Check sheet for the modelled part. Datum: model origin and axes. Units: mm. A direction names the side the tool comes from. Round coordinates to 2 decimals unless told otherwise and drop trailing zeros. Write each loop counter-clockwise with the first axis right and the second up, starting at its lowest first coordinate (ties: lowest second). Pieces come first, ordered by that corner, then holes.
from build123d import *

# Parameters (mm, degrees)
SKETCH_W             = 33
SKETCH_H             = 90.6
PAD_DEPTH            = 2
SKETCH001_W          = 31.55
SKETCH001_H          = 90.6
PAD001_DEPTH         = 14
SKETCH002_W          = 27.5
SKETCH002_H          = 72.5
POCKET_DEPTH         = 12.001
SKETCH003_W          = 19.5
SKETCH003_H          = 7.2
POCKET001_DEPTH      = 2.001
POCKET001_DEPTH_BACK = -12.001
SKETCH004_R          = 3.25
POCKET002_DEPTH      = 2
FILLET_R             = 2
FILLET001_R          = 1


with BuildPart() as part:
    # Sketch → Pad (new body)
    with BuildSketch(Plane.XY):
        with Locations((43.35, -0.5)):
            Rectangle(SKETCH_W, SKETCH_H)
    extrude(amount=PAD_DEPTH)

    # Sketch001 → Pad001 (join)
    with BuildSketch(Plane.XY):
        with Locations((44.075, -0.5)):
            Rectangle(SKETCH001_W, SKETCH001_H)
    extrude(amount=PAD001_DEPTH)

    # Sketch002 (on DatumPlane) → Pocket (cut, through all)
    with BuildSketch(Plane.XY.offset(2)):
        with Locations((44.05, 6.55)):
            Rectangle(SKETCH002_W, SKETCH002_H)
    extrude(amount=POCKET_DEPTH, mode=Mode.SUBTRACT)

    # Sketch003 (on DatumPlane) → Pocket001 (cut, two sides)
    with BuildSketch(Plane.XY.offset(2)) as pocket001_sk:
        with Locations((44.05, 46.4)):
            Rectangle(SKETCH003_W, SKETCH003_H)
    extrude(amount=-POCKET001_DEPTH, mode=Mode.SUBTRACT)
    extrude(pocket001_sk.sketch, amount=-POCKET001_DEPTH_BACK, mode=Mode.SUBTRACT)

    # Sketch004 → Pocket002 (cut)
    with BuildSketch(Plane.XY):
        with Locations((25, 39.5)):
            Circle(SKETCH004_R)
        with Locations((25, -39.5)):
            Circle(SKETCH004_R)
    extrude(amount=POCKET002_DEPTH, mode=Mode.SUBTRACT)

    # Fillet
    fillet_edges = [part.edges().sort_by_distance(p)[0] for p in [
        (43.35, -45.8, 0),
        (59.85, -0.5, 0),
        (56.825, 44.8, 0),
        (30.575, 44.8, 0),
        (59.85, -45.8, 7),
        (59.85, 44.8, 7),
    ]]
    fillet(fillet_edges, radius=FILLET_R)

    # Fillet001
    fillet001_edges = [part.edges().sort_by_distance(p)[0] for p in [
        (30.3, -29.7, 8),
        (57.8, -29.7, 8),
        (57.8, 42.8, 8),
        (30.3, 42.8, 8),
    ]]
    fillet(fillet001_edges, radius=FILLET001_R)


solid = part.part
1. Sectioned sample at D-D, the plane y = 39. Enter the section's corners in (x, z).
2. Release check for a two-part mould opening along X. For faces 4 (the cylindrical face through (28.25, 39.46, 0.99)), 5 (the flat face through (44, 7, 2)), 6 (the cylindrical face through (59.28, 44.2, 8.08)) record: released by +X, released by -X, zero draft, split by the parting line, or undercut.
3. Sectioned sample at C-C, the plane z = 3. Enter the section's corners in (x, y), plus the area to 3 significant figures.
4. Set-up check for faces 1 (the flat face through (59.85, -1, 8)), 2 (the flat face through (28.3, -1, 8)), 3 (the flat face through (30.3, 6, 8)): record each of +Z, -Z, +X, -X, +Y, -Y from which the full face is reachable in a straight line by a thin tool's end or side.
5. Sectioned sample at B-B, the plane x = 40. Enter the section's corners in (y, z), plus the area to 3 significant figures.
6. Go/stop test with flat-tipped pins: pin 1 (1.6 mm diameter, centred on x = 47.5, z = 1, fed in from +Y); pin 2 (0.6 mm diameter, centred on y = 44, z = 9.5, fed in from -X); pin 3 (8 mm diameter, centred on x = 54.5, y = 26, fed in from +Z); pin 4 (3.5 mm diameter, centred on x = 44, z = 8, fed in from +Y). Record where each tip stops, or that it passes through.
7. Scan lines: line 1 along X through (y, z) = (37, 13); line 2 along Y through (x, z) = (55, 7.25); line 3 along Z through (x, y) = (33, -21.5). Record each from-to range of solid material in increasing order.
8. Sectioned sample at A-A, the plane y = -27.5. Enter the section's corners in (x, z).
Computed values:
1. outline: (28.21, 0) - (57.85, 0) arc R2 ccw to (59.85, 2) - (59.85, 14) - (57.8, 14) - (57.8, 2) - (30.3, 2) - (30.3, 14) - (28.3, 14) - (28.3, 2) - (28.21, 2) - close
2. face 4: released by -X
2. face 5: undercut
2. face 6: released by +X
3. outline: (28.3, -45.8) - (57.85, -45.8) arc R2 ccw to (59.85, -43.8) - (59.85, 42.8) arc R2 ccw to (57.85, 44.8) - (53.8, 44.8) - (53.8, 42.8) - (56.8, 42.8) arc R1 cw to (57.8, 41.8) - (57.8, -28.7) arc R1 cw to (56.8, -29.7) - (31.3, -29.7) arc R1 cw to (30.3, -28.7) - (30.3, 41.8) arc R1 cw to (31.3, 42.8) - (34.3, 42.8) - (34.3, 44.8) - (28.3, 44.8) - close
3. area: 825 mm2
4. face 1: +Z, -Z, +X, +Y, -Y
4. face 2: +Z, -X, +Y, -Y
4. face 3: +Z
5. outline: (-45.8, 2) arc R2 ccw to (-43.8, 0) - (42.8, 0) - (42.8, 2) - (-29.7, 2) - (-29.7, 14) - (-45.8, 14) - close
5. area: 370 mm2
6. pin 1: stops at y = 42.8
6. pin 2: stops at x = 28.3
6. pin 3: stops at z = 14
6. pin 4: stops at y = -29.7
7. line 1: x = 28.3 to 30.3, 57.8 to 59.85
7. line 2: y = -45.8 to -29.7, 42.8 to 44.8
7. line 3: z = 0 to 2
8. outline: (26.85, 0) - (57.85, 0) arc R2 ccw to (59.85, 2) - (59.85, 14) - (57.8, 14) - (57.8, 2) - (30.3, 2) - (30.3, 14) - (28.3, 14) - (28.3, 2) - (26.85, 2) - close
